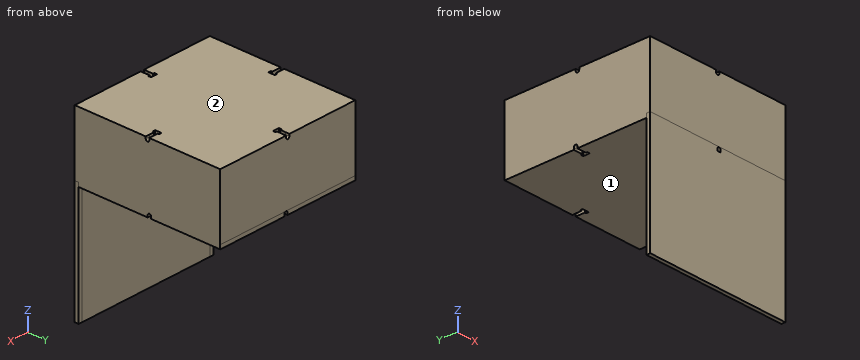
from build123d import *

# Parameters (mm, degrees)
SCHIZZO2_W                   = 123.3
SCHIZZO2_H                   = 123.3
ESTRUSIONE_ESTRUSIONE2_DEPTH = 53.3
SVUOTA1_T                    = -3.3
TAGLIO_ESTRUSIONE2_DEPTH     = 3.3
TAGLIO_ESTRUSIONE6_DEPTH     = 3.3
TAGLIO_ESTRUSIONE7_START     = 3.3
TAGLIO_ESTRUSIONE7_DEPTH     = 3.3
TAGLIO_ESTRUSIONE8_DEPTH     = 3.3
TAGLIO_ESTRUSIONE9_START     = -3.3
TAGLIO_ESTRUSIONE9_DEPTH     = 3.3
ESTRUSIONE_ESTRUSIONE5_DEPTH = 100
ESTRUSIONE_ESTRUSIONE7_DEPTH = 123.3
TAGLIO_ESTRUSIONE19_DEPTH    = 3.3
TAGLIO_ESTRUSIONE20_DEPTH    = 3.3
TAGLIO_ESTRUSIONE21_START    = -3.3
TAGLIO_ESTRUSIONE21_DEPTH    = 3.3
TAGLIO_ESTRUSIONE22_DEPTH    = 3.3
TAGLIO_ESTRUSIONE23_DEPTH    = 3.3
TAGLIO_ESTRUSIONE24_DEPTH    = 3.3


with BuildPart() as part:
    # Schizzo2 → Estrusione-Estrusione2 (new body)
    with BuildSketch(Plane.XY):
        with Locations((61.65, 61.65)):
            Rectangle(SCHIZZO2_W, SCHIZZO2_H)
    extrude(amount=-ESTRUSIONE_ESTRUSIONE2_DEPTH)

    # Svuota1
    svuota1_openings = [part.faces().sort_by_distance(p)[0] for p in [
        (61.65, 61.65, -53.3),
    ]]
    offset(amount=SVUOTA1_T, openings=svuota1_openings, kind=Kind.INTERSECTION)

    # Schizzo3D1 → Taglio-Estrusione2 (cut)
    with BuildSketch(Plane(origin=(123.3, 60.15, -1.65), x_dir=(0, 0.8762159086766463, 0.48191874977215726), z_dir=(1, 0, 0))):
        with BuildLine():
            Line((0, 0), (0.795165937, 1.445756249))
            Line((0.795165937, 1.445756249), (3.423813663, 0))
            Line((3.423813663, 0), (2.628647726, -1.445756249))
            ThreePointArc((2.628647726, -1.445756249), (0.591445738, -2.037201988), (0, 0))
        make_face()
    extrude(amount=-TAGLIO_ESTRUSIONE2_DEPTH, mode=Mode.SUBTRACT)

    # Schizzo6 → Taglio-Estrusione6 (cut)
    with BuildSketch(Plane.XY):
        Polygon((120, 60.15), (115.51, 60.15), (115.51, 58.92), (113.3, 58.92), (113.3, 64.38), (115.51, 64.38), (115.51, 63.15), (120, 63.15), align=None)
        Polygon((3.3, 63.15), (3.3, 60.15), (7.79, 60.15), (7.79, 58.92), (10, 58.92), (10, 64.38), (7.79, 64.38), (7.79, 63.15), align=None)
        Polygon((60.15, 3.3), (63.15, 3.3), (63.15, 7.79), (64.38, 7.79), (64.38, 10), (58.92, 10), (58.92, 7.79), (60.15, 7.79), align=None)
        Polygon((63.15, 120), (60.15, 120), (60.15, 115.51), (58.92, 115.51), (58.92, 113.3), (64.38, 113.3), (64.38, 115.51), (63.15, 115.51), align=None)
    extrude(amount=-TAGLIO_ESTRUSIONE6_DEPTH, mode=Mode.SUBTRACT)

    # Schizzo3D6 → Taglio-Estrusione7 (cut)
    with BuildSketch(Plane(origin=(0, 61.65, 0), x_dir=(0, -0.6726727939963129, -0.7399400733959435), z_dir=(1, 0, 0)).offset(TAGLIO_ESTRUSIONE7_START)):
        with BuildLine():
            Line((0, 0), (1.009009191, -1.10991011))
            Line((1.009009191, -1.10991011), (2.229910312, 0))
            ThreePointArc((2.229910312, 0), (2.321673153, 2.128880637), (0.192052014, 2.201454665))
            Line((0.192052014, 2.201454665), (-1.008845302, 1.109729832))
            Line((-1.008845302, 1.109729832), (0, 0))
        make_face()
    extrude(amount=-TAGLIO_ESTRUSIONE7_DEPTH, mode=Mode.SUBTRACT)

    # Schizzo3D7 → Taglio-Estrusione8 (cut)
    with BuildSketch(Plane(origin=(60.15, 0, 0), x_dir=(0.8760258326495893, 2.026216235651821e-15, -0.48226418126437076), z_dir=(0, -1, 0))):
        with BuildLine():
            Line((0, 0), (2.629562684, 1.447610159))
            Line((2.629562684, 1.447610159), (3.424555643, 0))
            ThreePointArc((3.424555643, 0), (2.832496055, -2.036456397), (0.795735899, -1.445442624))
            Line((0.795735899, -1.445442624), (0, 0))
        make_face()
    extrude(amount=-TAGLIO_ESTRUSIONE8_DEPTH, mode=Mode.SUBTRACT)

    # Schizzo3D8 → Taglio-Estrusione9 (cut)
    with BuildSketch(Plane(origin=(63.15, 123.3, 0), x_dir=(-0.8762159086766472, 0, -0.48191874977215554), z_dir=(0, 1, 0)).offset(TAGLIO_ESTRUSIONE9_START)):
        with BuildLine():
            Line((0, 0), (2.628647726, 1.445756249))
            Line((2.628647726, 1.445756249), (3.423813663, 0))
            ThreePointArc((3.423813663, 0), (2.832367925, -2.037201988), (0.795165937, -1.445756249))
            Line((0.795165937, -1.445756249), (0, 0))
        make_face()
    extrude(amount=TAGLIO_ESTRUSIONE9_DEPTH, mode=Mode.SUBTRACT)

    # Schizzo3D9 → Estrusione-Estrusione5 (add)
    with BuildSketch(Plane(origin=(120, 3.3, -53.3), x_dir=(-0.9996220893327035, -0.02748960745664935, 0), z_dir=(0, 0, 1))):
        Polygon((0, 0), (-3.298752895, 0.090715705), (-3.20803719, 3.389468599), (120.045366425, 0), (119.95465072, -3.298752895), (116.655897825, -3.20803719), align=None)
    extrude(amount=-ESTRUSIONE_ESTRUSIONE5_DEPTH)

    # Schizzo3D10 → Estrusione-Estrusione7 (add)
    with BuildSketch(Plane(origin=(123.3, 123.3, -53.3), x_dir=(0, -0.9996220893327035, -0.027489607456649322), z_dir=(-1, 0, 0))):
        Polygon((0, 0), (0.090715705, -3.298752895), (120.045366425, 0), (119.95465072, 3.298752895), align=None)
    extrude(amount=ESTRUSIONE_ESTRUSIONE7_DEPTH)

    # Schizzo14 → Taglio-Estrusione19 (cut)
    with BuildSketch(Plane.ZY):
        with BuildLine():
            Line((-56.6, 64.8), (-56.6, 61.8))
            Line((-56.6, 61.8), (-54.95, 61.8))
            ThreePointArc((-54.95, 61.8), (-53.45, 63.3), (-54.95, 64.8))
            Line((-54.95, 64.8), (-56.6, 64.8))
        make_face()
    extrude(amount=-TAGLIO_ESTRUSIONE19_DEPTH, mode=Mode.SUBTRACT)

    # Schizzo21 → Taglio-Estrusione20 (cut)
    with BuildSketch(Plane(origin=(0, 0, 0), x_dir=(-1, 0, 0), z_dir=(0, -1, 0))):
        with BuildLine():
            Line((-64.335889046, 56.848416793), (-64.335889046, 55.198416793))
            ThreePointArc((-64.335889046, 55.198416793), (-62.835889046, 53.698416793), (-61.335889046, 55.198416793))
            Line((-61.335889046, 55.198416793), (-61.335889046, 56.848416793))
            Line((-61.335889046, 56.848416793), (-64.335889046, 56.848416793))
        make_face()
    extrude(amount=-TAGLIO_ESTRUSIONE20_DEPTH, mode=Mode.SUBTRACT)

    # Schizzo17 → Taglio-Estrusione21 (cut)
    with BuildSketch(Plane(origin=(123.3, 0, 0), x_dir=(0, 0, -1), z_dir=(1, 0, 0)).offset(TAGLIO_ESTRUSIONE21_START)):
        with BuildLine():
            Line((56.6, 64.8), (56.6, 61.8))
            Line((56.6, 61.8), (54.95, 61.8))
            ThreePointArc((54.95, 61.8), (53.45, 63.3), (54.95, 64.8))
            Line((54.95, 64.8), (56.6, 64.8))
        make_face()
    extrude(amount=TAGLIO_ESTRUSIONE21_DEPTH, mode=Mode.SUBTRACT)

    # Schizzo24 → Taglio-Estrusione22 (cut)
    with BuildSketch(Plane(origin=(0, 123.3, 0), x_dir=(1, 0, 0), z_dir=(0, 1, 0))):
        with BuildLine():
            Line((61.734441738, 56.603992056), (61.734441738, 54.953992056))
            ThreePointArc((61.734441738, 54.953992056), (63.234441738, 53.453992056), (64.734441738, 54.953992056))
            Line((64.734441738, 54.953992056), (64.734441738, 56.603992056))
            Line((64.734441738, 56.603992056), (61.734441738, 56.603992056))
        make_face()
    extrude(amount=-TAGLIO_ESTRUSIONE22_DEPTH, mode=Mode.SUBTRACT)

    # Schizzo26 → Taglio-Estrusione23 (cut)
    with BuildSketch(Plane(origin=(0, 0, -56.6), x_dir=(-1, 0, 0), z_dir=(0, 0, -1))):
        Polygon((-61.734441738, 120), (-61.734441738, 115.51), (-60.504441738, 115.51), (-60.504441738, 113.3), (-65.964441738, 113.3), (-65.964441738, 115.51), (-64.734441738, 115.51), (-64.734441738, 120), align=None)
    extrude(amount=-TAGLIO_ESTRUSIONE23_DEPTH, mode=Mode.SUBTRACT)

    # Schizzo28 → Taglio-Estrusione24 (cut)
    with BuildSketch(Plane(origin=(0, 0, -56.6), x_dir=(-1, 0, 0), z_dir=(0, 0, -1))):
        Polygon((-120, 61.8), (-115.51, 61.8), (-115.51, 60.57), (-113.3, 60.57), (-113.3, 66.03), (-115.51, 66.03), (-115.51, 64.8), (-120, 64.8), align=None)
        Polygon((-3.3, 64.8), (-7.79, 64.8), (-7.79, 66.03), (-10, 66.03), (-10, 60.57), (-7.79, 60.57), (-7.79, 61.8), (-3.3, 61.8), align=None)
        Polygon((-64.335889046, 3.3), (-64.335889046, 7.79), (-65.565889046, 7.79), (-65.565889046, 10), (-60.105889046, 10), (-60.105889046, 7.79), (-61.335889046, 7.79), (-61.335889046, 3.3), align=None)
    extrude(amount=-TAGLIO_ESTRUSIONE24_DEPTH, mode=Mode.SUBTRACT)


solid = part.part
Here's how the part is built. I have some questions about the finished solid (model axes, mm). Face numbers are marked on the shaded views. A direction names the side the tool comes from. Coordinates: 2 decimals unless noted, no trailing zeros. Order: outer loops, then holes, each group sorted by start corner. A loop starts at its lowest first (then second) coordinate and runs counter-clockwise, first axis right, second up. Notation, with made-up numbers: (89, -36) - (135, -36) arc R3 ccw to (135, -31) - close; hole circle Ø6 at (7, -26). An arc over 180 degrees is marked (long way). Use CSV: the item, a comma, the result in double quotes. Start each with the question number.
1. Suppose I cut it at C-C on z = -124.5. List the corners of the cut face in (x, y) for me, then the cut area to 3 significant figures.
2. Suppose I cut it at A-A on z = -26.5. List the corners of the cut face in (x, y) for me, then the cut area to 3 significant figures.
3. I'm going to push flat-ended pins straight in: pin 1 (1.4 mm diameter, centred on y = 59.5, z = -1.5, fed in from -X); pin 2 (12 mm diameter, centred on x = 66, y = 25, fed in from -Z); pin 3 (1 mm diameter, centred on x = 121.5, z = -97.5, fed in from +Y). Where does each tip first touch, or does it pass through?
4. Suppose I cut it at B-B on x = 84. List the corners of the cut face in (y, z) for me.
5. For the marked faces 1 and 2, which set-ups out of +Z, -Z, +X, -X, +Y, -Y let a thin tool reach every point of the face, with its end or its side?
6. Please list where these lines run through material, in increasing order: line 1 (Z direction, x = 18.5, y = 75.5); line 2 (Y direction, x = 8, z = -26). Write a range as from..to.
Output:
1,outline,"(0, 0) - (123.3, 0) - (123.3, 3.3) - (0, 3.3) - close"
1,area,"407 mm2"
2,outline,"(0, 0) - (123.3, 0) - (123.3, 123.3) - (0, 123.3) - close; hole (3.3, 3.3) - (120, 3.3) - (120, 120) - (3.3, 120) - close"
2,area,"1,580 mm2"
3,pin 1,"stops at x = 0"
3,pin 2,"stops at z = -56.6"
3,pin 3,"stops at y = 3.3"
4,outline,"(0, -153.3) - (3.3, -153.3) - (3.3, -56.6) - (123.3, -56.6) - (123.3, 0) - (0, 0) - close; hole (3.3, -53.3) - (120, -53.3) - (120, -3.3) - (3.3, -3.3) - close"
5,face 1,"-Z, +X, -X, +Y"
5,face 2,"+Z, +X, -X, +Y, -Y"
6,line 1,"z = -56.6..-53.3, -3.3..0"
6,line 2,"y = 0..3.3, 120..123.3"
